```python
from build123d import *

# Parameters (mm, degrees)
SKETCH_1_W          = 60
SKETCH_1_H          = 35.8
EXTRUDE_1_DEPTH     = 30
SKETCH_2_W          = 50.4
SKETCH_2_H          = 18.4
CUT_EXTRUDE_1_DEPTH = 47.047909833
CHAMFER_1_SIZE      = 2
CHAMFER_1_SIZE2     = 11.342563639
CHAMFER_2_SIZE      = 2


with BuildPart() as part:
    # 草图1 → 凸台-拉伸1 (new body)
    with BuildSketch(Plane.XY):
        Rectangle(SKETCH_1_W, SKETCH_1_H)
    extrude(amount=EXTRUDE_1_DEPTH)

    # 草图2 → 切除-拉伸1 (cut, through all)
    with BuildSketch(Plane.XY.offset(30)):
        Rectangle(SKETCH_2_W, SKETCH_2_H)
    extrude(amount=-CUT_EXTRUDE_1_DEPTH, mode=Mode.SUBTRACT)

    # 倒角1
    chamfer_1_edges = [part.edges().sort_by_distance(p)[0] for p in [
        (30, -17.9, 15),
        (30, 17.9, 15),
    ]]
    chamfer_1_side = [part.faces().sort_by_distance(p)[0] for p in [
        (30, 0, 15),
    ]]
    chamfer(chamfer_1_edges, length=CHAMFER_1_SIZE, length2=CHAMFER_1_SIZE2, reference=chamfer_1_side[0])

    # 倒角2
    chamfer_2_edges = [part.edges().sort_by_distance(p)[0] for p in [
        (0, 9.2, 30),
        (-25.2, 0, 30),
        (0, -9.2, 30),
        (30, 0, 30),
    ]]
    chamfer(chamfer_2_edges, length=CHAMFER_2_SIZE)


solid = part.part
```
Can you work these out from the model? Positions are in its coordinate system, mm. A direction names the side the tool comes from. Coordinates: 2 decimals unless noted, no trailing zeros. Loops run counter-clockwise (first coordinate to the right, second up) from the corner with the lowest first, then second, coordinate; pieces in that order, holes last.
1) Thinking about a two-plate mould opening in Y: for faces 1 (the flat face through (-6, 17.9, 15)), 2 (the flat face through (29, 0, 29)), 3 (the flat face through (25.2, 0, 15)), which applies, pulls with the +Y half, pulls with the -Y half, needs draft (parallel to the pull), parting line crosses it, or undercut?
2) Imagine slicing it at D-D on x = -26. List the corners of the cut face in (y, z) for me, plus the area to 3 significant figures.
3) Imagine slicing it at A-A on z = 12.5. List the corners of the cut face in (x, y) for me.
4) Imagine slicing it at B-B on y = 2. List the corners of the cut face in (x, z) for me, plus the area to 3 significant figures.
5) Which directions (+Z, -Z, +X, -X, +Y, -Y) give clear straight access to the entire face, cutting with the end or side of a thin tool? Please do faces 4 (the flat face through (-25.2, 0, 14)), 5 (the flat face through (30, 0, 14)), 6 (the flat face through (-26.2, -0.2, 29)).
6) Imagine slicing it at C-C on x = 11. List the corners of the cut face in (y, z) for me.
7) I need wall thicknesses on probe 1 along Y at (x, z) = (5, 15.5); probe 2 along X at (y, z) = (-1, 21); probe 3 along Z at (x, y) = (13, 11). Which ranges of each line are inside material? Lowest first, please.
8) For pin 1 (12 mm diameter, centred on x = -15, y = -2.5, fed in from -Z), with a flat end and sliding along its axis, tell me the tip position at first contact or that it passes through.
Completed:
1. face 1: pulls with the +Y half
1. face 2: needs draft
1. face 3: undercut
2. outline: (-17.9, 0) - (17.9, 0) - (17.9, 30) - (11.2, 30) - (10, 28.8) - (-10, 28.8) - (-11.2, 30) - (-17.9, 30) - close
2. area: 1,050 mm2
3. outline: (-30, -17.9) - (18.66, -17.9) - (30, -15.9) - (30, 15.9) - (18.66, 17.9) - (-30, 17.9) - close; hole (-25.2, -9.2) - (25.2, -9.2) - (25.2, 9.2) - (-25.2, 9.2) - close
4. outline: (-30, 0) - (-25.2, 0) - (-25.2, 28) - (-27.2, 30) - (-30, 30) - close; (25.2, 0) - (30, 0) - (30, 28) - (28, 30) - (25.2, 30) - close
4. area: 284 mm2
5. face 4: +Z, -Z
5. face 5: +Z, -Z, +X, +Y, -Y
5. face 6: +Z
6. outline: (-17.9, 0) - (-9.2, 0) - (-9.2, 28) - (-11.2, 30) - (-17.9, 30) - close; (9.2, 0) - (17.9, 0) - (17.9, 30) - (11.2, 30) - (9.2, 28) - close
7. probe 1: y = -17.9 to -9.2, 9.2 to 17.9
7. probe 2: x = -30 to -25.2, 25.2 to 30
7. probe 3: z = 0 to 29.8
8. pin 1: passes through
